from build123d import *

# Parameters (mm, degrees)
PAD_DEPTH       = 2
PAD001_DEPTH    = 3
PAD002_DEPTH    = 1.2
SKETCH004_W     = 8.8
SKETCH004_H     = 3
POCKET_DEPTH    = 2
SKETCH005_W     = 3.5
SKETCH005_H     = 9.2
POCKET001_DEPTH = 2
SKETCH006_W     = 10
SKETCH006_H     = 5
POCKET002_DEPTH = 2
CHAMFER_SIZE    = 0.5
SKETCH007_W     = 3
SKETCH007_H     = 0.4
PAD003_DEPTH    = 0.3
SKETCH008_W     = 1
SKETCH008_H     = 1.2
POCKET003_DEPTH = 1
FILLET_R        = 0.199
SKETCH009_W     = 3
SKETCH009_H     = 0.4
PAD004_DEPTH    = 0.3
FILLET001_R     = 0.19
SKETCH010_W     = 1
SKETCH010_H     = 1.2
POCKET004_DEPTH = 1
FILLET002_R     = 0.5
SKETCH011_W     = 4.9
SKETCH011_H     = 1
PAD005_DEPTH    = 3.1


with BuildPart() as part:
    # Sketch → Pad (new body)
    with BuildSketch(Plane.XY):
        with BuildLine():
            Line((-21.8, -11.3), (21.8, -11.3))
            ThreePointArc((21.8, -11.3), (23.214214, -10.714214), (23.8, -9.3))
            Line((23.8, -9.3), (23.8, 9.3))
            ThreePointArc((23.8, 9.3), (23.214214, 10.714214), (21.8, 11.3))
            Line((21.8, 11.3), (-21.8, 11.3))
            ThreePointArc((-21.8, 11.3), (-23.214214, 10.714214), (-23.8, 9.3))
            Line((-23.8, 9.3), (-23.8, -9.3))
            ThreePointArc((-23.8, -9.3), (-23.214214, -10.714214), (-21.8, -11.3))
        make_face()
    extrude(amount=PAD_DEPTH)

    # Sketch002 (on Face9 of Pad) → Pad001 (join)
    with BuildSketch(Plane(origin=(0, 0, 0), x_dir=(1, 0, 0), z_dir=(0, 0, -1))):
        with BuildLine():
            Line((-23.8, 9.3), (-23.8, -9.3))
            ThreePointArc((-23.8, -9.3), (-23.214214, -10.714214), (-21.8, -11.3))
            Line((-21.8, -11.3), (21.8, -11.3))
            ThreePointArc((21.8, -11.3), (23.214214, -10.714214), (23.8, -9.3))
            Line((23.8, -9.3), (23.8, 9.3))
            ThreePointArc((23.8, 9.3), (23.214214, 10.714214), (21.8, 11.3))
            Line((21.8, 11.3), (-21.8, 11.3))
            ThreePointArc((-21.8, 11.3), (-23.214214, 10.714214), (-23.8, 9.3))
        make_face()
        with BuildLine():
            Line((-21.8, 8.3), (-21.8, -8.3))
            ThreePointArc((-21.8, -8.3), (-21.507107, -9.007107), (-20.8, -9.3))
            Line((-20.8, -9.3), (20.8, -9.3))
            ThreePointArc((20.8, -9.3), (21.507107, -9.007107), (21.8, -8.3))
            Line((21.8, -8.3), (21.8, 8.3))
            ThreePointArc((21.8, 8.3), (21.507107, 9.007107), (20.8, 9.3))
            Line((20.8, 9.3), (-20.8, 9.3))
            ThreePointArc((-20.8, 9.3), (-21.507107, 9.007107), (-21.8, 8.3))
        make_face(mode=Mode.SUBTRACT)
    extrude(amount=PAD001_DEPTH)

    # Sketch003 (on Face1 of Pad001) → Pad002 (join)
    with BuildSketch(Plane(origin=(0, 0, -3), x_dir=(1, 0, 0), z_dir=(0, 0, -1))):
        with BuildLine():
            Line((-22.75, 9.273817), (-22.75, -8.811393))
            ThreePointArc((-22.75, -8.811393), (-22.328642, -9.828642), (-21.311393, -10.25))
            Line((-21.311393, -10.25), (20.79762, -10.25))
            ThreePointArc((20.79762, -10.25), (22.178161, -9.678161), (22.75, -8.29762))
            Line((22.75, -8.29762), (22.75, 8.43735))
            ThreePointArc((22.75, 8.43735), (22.219087, 9.719087), (20.93735, 10.25))
            Line((20.93735, 10.25), (-21.773817, 10.25))
            ThreePointArc((-21.773817, 10.25), (-22.464083, 9.964083), (-22.75, 9.273817))
        make_face()
        with BuildLine():
            Line((-21.8, 8.3), (-21.8, -8.3))
            ThreePointArc((-21.8, -8.3), (-21.507107, -9.007107), (-20.8, -9.3))
            Line((-20.8, -9.3), (20.8, -9.3))
            ThreePointArc((20.8, -9.3), (21.507107, -9.007107), (21.8, -8.3))
            Line((21.8, -8.3), (21.8, 8.3))
            ThreePointArc((21.8, 8.3), (21.507107, 9.007107), (20.8, 9.3))
            Line((20.8, 9.3), (-20.8, 9.3))
            ThreePointArc((-20.8, 9.3), (-21.507107, 9.007107), (-21.8, 8.3))
        make_face(mode=Mode.SUBTRACT)
    extrude(amount=PAD002_DEPTH)

    # Sketch004 (on Face2 of Pad002) → Pocket (cut)
    with BuildSketch(Plane(origin=(-23.8, 0, 0), x_dir=(0, -1, 0), z_dir=(-1, 0, 0))):
        with Locations((1.797054, -2.857067)):
            Rectangle(SKETCH004_W, SKETCH004_H)
    extrude(amount=-POCKET_DEPTH, mode=Mode.SUBTRACT)

    # Sketch005 (on Face21 of Pocket) → Pocket001 (cut)
    with BuildSketch(Plane.XY.offset(2)):
        with Locations((18.75, -2.9)):
            Rectangle(SKETCH005_W, SKETCH005_H)
    extrude(amount=-POCKET001_DEPTH, mode=Mode.SUBTRACT)

    # Sketch006 (on Face15 of Pocket001) → Pocket002 (cut)
    with BuildSketch(Plane(origin=(0, 11.3, 0), x_dir=(-1, 0, 0), z_dir=(0, 1, 0))):
        with Locations((-16, -2.5)):
            Rectangle(SKETCH006_W, SKETCH006_H)
    extrude(amount=-POCKET002_DEPTH, mode=Mode.SUBTRACT)

    # Chamfer
    chamfer_edges = [part.edges().sort_by_distance(p)[0] for p in [
        (-23.8, 2.602946, -2.178533),
        (-23.8, -1.797054, -1.357067),
        (-23.8, -6.197054, -2.178533),
    ]]
    chamfer(chamfer_edges, length=CHAMFER_SIZE)

    # Sketch007 (on Face11 of Chamfer) → Pad003 (join)
    with BuildSketch(Plane.XZ.offset(10.25)):
        with Locations((-15.273817, -4)):
            Rectangle(SKETCH007_W, SKETCH007_H)
        with Locations((14.43735, -4)):
            Rectangle(SKETCH007_W, SKETCH007_H)
    extrude(amount=PAD003_DEPTH)

    # Sketch008 (on Face11 of Pad003) → Pocket003 (cut)
    with BuildSketch(Plane.XZ.offset(10.25)):
        with Locations((-17.273817, -3.6)):
            Rectangle(SKETCH008_W, SKETCH008_H)
        with Locations((-13.273817, -3.6)):
            Rectangle(SKETCH008_W, SKETCH008_H)
        with Locations((16.43735, -3.6)):
            Rectangle(SKETCH008_W, SKETCH008_H)
        with Locations((12.43735, -3.6)):
            Rectangle(SKETCH008_W, SKETCH008_H)
    extrude(amount=-POCKET003_DEPTH, mode=Mode.SUBTRACT)

    # Fillet
    fillet_edges = [part.edges().sort_by_distance(p)[0] for p in [
        (-15.273817, -10.55, -3.8),
        (-15.273817, -10.55, -4.2),
        (14.43735, -10.55, -3.8),
        (14.43735, -10.55, -4.2),
    ]]
    fillet(fillet_edges, radius=FILLET_R)

    # Sketch009 (on Face65 of Fillet) → Pad004 (join)
    with BuildSketch(Plane(origin=(0, 10.25, 0), x_dir=(-1, 0, 0), z_dir=(0, 1, 0))):
        with Locations((15.3, -4)):
            Rectangle(SKETCH009_W, SKETCH009_H)
        with Locations((-6.5, -4)):
            Rectangle(SKETCH009_W, SKETCH009_H)
    extrude(amount=PAD004_DEPTH)

    # Fillet001
    fillet001_edges = [part.edges().sort_by_distance(p)[0] for p in [
        (6.5, 10.55, -3.8),
        (6.5, 10.55, -4.2),
        (-15.3, 10.55, -3.8),
        (-15.3, 10.55, -4.2),
    ]]
    fillet(fillet001_edges, radius=FILLET001_R)

    # Sketch010 (on Face4 of Fillet001) → Pocket004 (cut)
    with BuildSketch(Plane(origin=(0, 10.25, 0), x_dir=(-1, 0, 0), z_dir=(0, 1, 0))):
        with Locations((-8.5, -3.6)):
            Rectangle(SKETCH010_W, SKETCH010_H)
        with Locations((-4.5, -3.6)):
            Rectangle(SKETCH010_W, SKETCH010_H)
        with Locations((13.3, -3.6)):
            Rectangle(SKETCH010_W, SKETCH010_H)
        with Locations((17.3, -3.6)):
            Rectangle(SKETCH010_W, SKETCH010_H)
    extrude(amount=-POCKET004_DEPTH, mode=Mode.SUBTRACT)

    # Fillet002
    fillet002_edges = [part.edges().sort_by_distance(p)[0] for p in [
        (23.8, 0, 2),
        (23.214214, 10.714214, 2),
        (0, 11.3, 2),
        (-23.214214, 10.714214, 2),
        (-23.8, 0, 2),
        (-23.214214, -10.714214, 2),
        (0, -11.3, 2),
        (23.214214, -10.714214, 2),
    ]]
    fillet(fillet002_edges, radius=FILLET002_R)

    # Sketch011 (on Face4 of Fillet002) → Pad005 (join)
    with BuildSketch(Plane(origin=(0, 0, -3), x_dir=(1, 0, 0), z_dir=(0, 0, -1))):
        with Locations((1.2, 10.75)):
            Rectangle(SKETCH011_W, SKETCH011_H)
    extrude(amount=PAD005_DEPTH)


solid = part.part
For this review, take the finished solid that the model builds, in its own axes (mm). A direction names the side the tool comes from. Round coordinates to 2 decimals unless told otherwise and drop trailing zeros. Write each loop counter-clockwise with the first axis right and the second up, starting at its lowest first coordinate (ties: lowest second). Pieces come first, ordered by that corner, then holes. Notation, with made-up numbers: M 77.5,69 L 119.5,69 A10 ccw 119.5,76 Z; hole C -37.75,-9 d3. An arc over 180 degrees is marked long. Write item = value, one per line. Start each with the question number.
(1) The part is to be moulded in two halves that separate along X. For faces 4 (the face through (-22.34, 9.82, -3.59)), 5 (the face through (12.937, -10, -4)), 6 (the face through (-15, 10, -4.2)), say which applies: +X half, -X half, draft (parallel to the pull), parting line (faces both ways), or undercut.
(2) For line 1 along Y through (x, z) = (18, 1.5); line 2 along Y through (x, z) = (6.5, -2.5); line 3 along Z through (x, y) = (4, 5.25), list the stretches that pass through material, from the lowest coordinate up.
(3) We need section B-B (z = -2.25). Give the boundary of the cut face in (x, y).
(4) For faces 1 (the face through (-7, -10.25, -4)), 2 (the face through (9, 10, -4)), 3 (the face through (19, 1.7, 1)), list the 3-axis set-ups (+Z, -Z, +X, -X, +Y, -Y) from which the entire face can be reached by the end or side of a thin tool; tool diameter is ignored.
(5) Clearance check with flat-ended pins moving along their axes: pin 1 Ø0.5 at (y, z) = (10, -3.5) entering from +X; pin 2 Ø1 at (x, y) = (-0.5, 6) entering from -Z; pin 3 Ø0.9 at (x, z) = (6.5, -3.5) entering from +Y. State where each tip first meets the part, or that it passes through.
(6) We need section A-A (y = -5.75). Give the boundary of the cut face in (x, z).
(7) We need section D-D (z = 1). Give the boundary of the cut face in (x, y), then the cut area to 3 significant figures.
Results found:
q1.face_4 = -X half
q1.face_5 = undercut
q1.face_6 = draft
q2.line_1 = -11.3 to -7.5, 1.7 to 11.3
q2.line_2 = -11.3 to -9.3, 9.3 to 11.3
q2.line_3 = 0 to 2
q3.outline = M -23.8,-9.3 A2 ccw -21.8,-11.3 L 21.8,-11.3 A2 ccw 23.8,-9.3 L 23.8,9.3 A2 ccw 21.8,11.3 L 21,11.3 L 21,9.3 L 20.8,9.3 A1 cw 21.8,8.3 L 21.8,-8.3 A1 cw 20.8,-9.3 L -20.8,-9.3 A1 cw -21.8,-8.3 L -21.8,-6.2 L -23.3,-6.2 L -23.8,-6.7 Z; M -23.8,3.1 L -23.3,2.6 L -21.8,2.6 L -21.8,8.3 A1 cw -20.8,9.3 L 11,9.3 L 11,11.3 L -21.8,11.3 A2 ccw -23.8,9.3 Z
q4.face_1 = -Z, -Y
q4.face_2 = -Z, +Y
q4.face_3 = +Z, -Z
q5.pin_1 = 22.1
q5.pin_2 = 0
q5.pin_3 = 10.55
q6.outline = M -23.8,-0.86 L -23.3,-1.36 L -21.8,-1.36 L -21.8,0 L 17,0 L 17,2 L -23.3,2 A0.5 ccw -23.8,1.5 Z; M 20.5,0 L 21.8,0 L 21.8,-4.2 L 22.75,-4.2 L 22.75,-3 L 23.8,-3 L 23.8,1.5 A0.5 ccw 23.3,2 L 20.5,2 Z
q7.outline = M -23.8,-9.3 A2 ccw -21.8,-11.3 L 21.8,-11.3 A2 ccw 23.8,-9.3 L 23.8,9.3 A2 ccw 21.8,11.3 L -21.8,11.3 A2 ccw -23.8,9.3 Z; hole M 17,-7.5 L 20.5,-7.5 L 20.5,1.7 L 17,1.7 Z
q7.area = 1,040 mm²
